```python
from build123d import *

# Parameters (mm, degrees)
SKETCH_1_R          = 1.354010502
EXTRUDE_1_DEPTH     = 3
SKETCH_2_R          = 1.6
CUT_EXTRUDE_1_DEPTH = 61.466769186


with BuildPart() as part:
    # 草图1 → 凸台-拉伸1 (new body)
    with BuildSketch(Plane(origin=(0, 0, 0), x_dir=(-1, 0, 0), z_dir=(0, 0, -1))):
        with BuildLine():
            Line((-55.860221974, 0), (24.13832066, 0))
            ThreePointArc((24.13832066, 0), (26.966394209, 1.171219344), (28.138320535, 3.999))
            ThreePointArc((28.138320535, 3.999), (26.96674766, 6.827427125), (24.138320535, 7.999))
            Line((24.138320535, 7.999), (-55.860222099, 7.999))
            ThreePointArc((-55.860222099, 7.999), (-58.688295648, 6.827780656), (-59.860221974, 4))
            ThreePointArc((-59.860221974, 4), (-58.688649099, 1.171572875), (-55.860221974, 0))
        make_face()
        with Locations((24.138809001, 3.998511534)):
            Circle(SKETCH_1_R, mode=Mode.SUBTRACT)
        with Locations((-55.859733508, 3.999511534)):
            Circle(SKETCH_1_R, mode=Mode.SUBTRACT)
    extrude(amount=-EXTRUDE_1_DEPTH)

    # 草图2 → 切除-拉伸1 (cut, through all)
    with BuildSketch(Plane.XY.offset(3)):
        with Locations((-24.138809001, 3.998511534)):
            Circle(SKETCH_2_R)
    extrude(amount=-CUT_EXTRUDE_1_DEPTH, mode=Mode.SUBTRACT)


solid = part.part
```
Geometry: final body of the model. Coordinates: model frame, mm. Coordinates: 2 decimals unless noted, no trailing zeros. Loops run counter-clockwise (first coordinate to the right, second up) from the corner with the lowest first, then second, coordinate; pieces in that order, holes last. Notation, with made-up numbers: M 2.25,38 L 19.25,38 A21 ccw 19.25,55 Z; hole C 42.5,34.25 d2. An arc over 180 degrees is marked long. Put each result on its own line as item: value.
(1) Cut plane A-A on z = 0.6. Return the cut outline in (x, y), then the cut area to 3 significant figures.
Answer sheet:
outline: M -28.14,4 A4 ccw -24.14,0 L 55.86,0 A4 ccw 59.86,4 A4 ccw 55.86,8 L -24.14,8 A4 ccw Z; hole C -24.14,4 d3.2; hole C 55.86,4 d2.71
area: 676 mm^2
(2) Draft query along X for faces 1 (the face through (56.934, 3.176, 1.479)), 2 (the face through (16, 4, 3)). Return one class per face: pulls with the +X half, pulls with the -X half, needs draft (parallel to the pull), parting line crosses it, or undercut.
Answer sheet:
face 1: undercut
face 2: needs draft
(3) Cut plane B-B on y = 6.75. Return the cut outline in (x, z).
Answer sheet:
outline: M -27.04,0 L 58.76,0 L 58.76,3 L -27.04,3 Z
(4) Material intervals for probe 1 along X at (y, z) = (5, 0.8); probe 2 along X at (y, z) = (3.75, 1.85); probe 3 along Y at (x, z) = (55, 1.4), sorted ascending.
Answer sheet:
probe 1: x = -28.01 to -25.39, -22.89 to 54.95, 56.77 to 59.73
probe 2: x = -28.13 to -25.72, -22.56 to 54.53, 57.19 to 59.85
probe 3: y = 0 to 2.95, 5.05 to 8
(5) First-contact query: pin 1 (4.5 mm diameter, centred on x = 55.86, y = 4, fed in from -Z); pin 2 (1 mm diameter, centred on y = 5.5, z = 1, fed in from -X). Flat tips, straight axial feed; report the tip coordinate or a pass-through.
Answer sheet:
pin 1: stops at z = 0
pin 2: stops at x = -28.01
